Read the model definition and answer for the solid it produces. Units are mm, in the model's axes. Face numbers are marked on the shaded views. A direction names the side the tool comes from. Coordinates: 2 decimals unless noted, no trailing zeros. Loops run counter-clockwise (first coordinate to the right, second up) from the corner with the lowest first, then second, coordinate; pieces in that order, holes last.
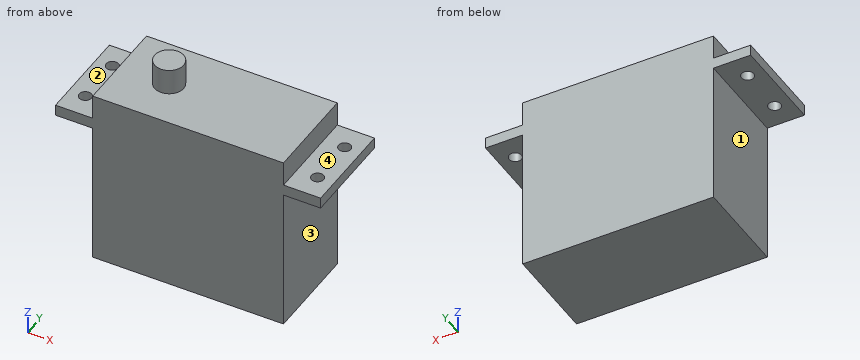
from build123d import *

# Parameters (mm, degrees)
SKETCH1_W                        = 54.356
SKETCH1_H                        = 19.685
EXTRUDE1_DEPTH                   = 42.2656
SKETCH3_OUTSIDE_W                = 70.678
SKETCH3_OUTSIDE_H                = 36.007
SKETCH3_OUTSIDE_R                = 2.9718
EXTRUDE2_DEPTH                   = 5.334
SKETCH7_W                        = 7.62
SKETCH7_H                        = 20.335773086
SKETCH7_H_2                      = 19.919316746
EXTRUDE4_DEPTH                   = 10.414
SKETCH8_W                        = 7.62
SKETCH8_H                        = 19.792977092
SKETCH8_H_2                      = 19.986836906
EXTRUDE5_DEPTH                   = 29.5656
F_39_0_0995_DIAMETER_HOLE1_D     = 2.5273
F_39_0_0995_DIAMETER_HOLE1_DEPTH = 12.7
F_39_0_0995_DIAMETER_HOLE1_TIP   = 0.759277521


with BuildPart() as part:
    # Sketch1 → Extrude1 (new body)
    with BuildSketch(Plane.XY):
        Rectangle(SKETCH1_W, SKETCH1_H)
    extrude(amount=EXTRUDE1_DEPTH)

    # Sketch3 outside → Extrude2 (cut)
    with BuildSketch(Plane.XY.offset(42.2656)):
        with Locations((0, 0.0005)):
            Rectangle(SKETCH3_OUTSIDE_W, SKETCH3_OUTSIDE_H)
        with Locations((-9.398, 0)):
            Circle(SKETCH3_OUTSIDE_R, mode=Mode.SUBTRACT)
    extrude(amount=-EXTRUDE2_DEPTH, mode=Mode.SUBTRACT)

    # Sketch7 → Extrude4 (cut)
    with BuildSketch(Plane.XY.offset(42.2656)):
        with Locations((23.368, 0)):
            Rectangle(SKETCH7_W, SKETCH7_H)
        with Locations((-23.368, 0)):
            Rectangle(SKETCH7_W, SKETCH7_H_2)
    extrude(amount=-EXTRUDE4_DEPTH, mode=Mode.SUBTRACT)

    # Sketch8 → Extrude5 (cut)
    with BuildSketch(Plane(origin=(0, 0, 0), x_dir=(-1, 0, 0), z_dir=(0, 0, -1))):
        with Locations((23.368, 0)):
            Rectangle(SKETCH8_W, SKETCH8_H)
        with Locations((-23.368, 0)):
            Rectangle(SKETCH8_W, SKETCH8_H_2)
    extrude(amount=-EXTRUDE5_DEPTH, mode=Mode.SUBTRACT)

    # #39 (0.0995) Diameter Hole1
    with Locations(Plane(origin=(-23.8125, 4.953, 31.8516), x_dir=(1, 0, 0), z_dir=(0, 0, 1))):
        with Locations((0, 0), (0, -9.906), (47.625, 0), (47.625, -9.906)):
            Hole(F_39_0_0995_DIAMETER_HOLE1_D / 2, depth=F_39_0_0995_DIAMETER_HOLE1_DEPTH)
            with Locations((0, 0, -(F_39_0_0995_DIAMETER_HOLE1_DEPTH + F_39_0_0995_DIAMETER_HOLE1_TIP / 2))):  # 118° drill point
                Cone(0, F_39_0_0995_DIAMETER_HOLE1_D / 2, F_39_0_0995_DIAMETER_HOLE1_TIP, mode=Mode.SUBTRACT)


solid = part.part
Q1. A cutting plane is placed at D-D (y = 7). Give the vertices of the cut face in (x, z).
Findings below:
outline: (-27.18, 29.57) - (-19.56, 29.57) - (-19.56, 0) - (19.56, 0) - (19.56, 29.57) - (27.18, 29.57) - (27.18, 31.85) - (19.56, 31.85) - (19.56, 36.93) - (-19.56, 36.93) - (-19.56, 31.85) - (-27.18, 31.85) - close
Q2. Which of the six approach directions +Z, -Z, +X, -X, +Y, -Y give full straight-line access (tool end or side, diameter ignored) to the marked faces 1, 2, 3 and 4?
Findings below:
face 1: -Z, -X, +Y, -Y
face 2: +Z, -X, +Y, -Y
face 3: -Z, +X, +Y, -Y
face 4: +Z, +X, +Y, -Y
Q3. Flat-ended cylindrical pins translate along their axes: pin 1 Ø1 at (y, z) = (-4.5, 35) entering from +X; pin 2 Ø3 at (x, y) = (-23.81, -4.95) entering from +Z; pin 3 Ø6 at (x, y) = (6.5, -3) entering from +Z. Find the tip coordinate at first contact, or state that the pin passes through.
Findings below:
pin 1: stops at x = 19.56
pin 2: stops at z = 31.85
pin 3: stops at z = 36.93
Q4. A cutting plane is placed at A-A (x = 23.5). Give the vertices of the cut face in (y, z), then the cut area to 3 significant figures.
Findings below:
outline: (-9.84, 29.57) - (-6.18, 29.57) - (-6.18, 31.85) - (-9.84, 31.85) - close; (-3.73, 29.57) - (3.73, 29.57) - (3.73, 31.85) - (-3.73, 31.85) - close; (6.18, 29.57) - (9.84, 29.57) - (9.84, 31.85) - (6.18, 31.85) - close
area: 33.8 mm2
Q5. A cutting plane is placed at B-B (y = 0). Give the vertices of the cut face in (x, z).
Findings below:
outline: (-27.18, 29.57) - (-19.56, 29.57) - (-19.56, 0) - (19.56, 0) - (19.56, 29.57) - (27.18, 29.57) - (27.18, 31.85) - (19.56, 31.85) - (19.56, 36.93) - (-6.43, 36.93) - (-6.43, 42.27) - (-12.37, 42.27) - (-12.37, 36.93) - (-19.56, 36.93) - (-19.56, 31.85) - (-27.18, 31.85) - close
Q6. Straight lines are drawn through the part: probe 1 along Z at (x, y) = (8, 2.5); probe 2 along X at (y, z) = (8.25, 10.5); probe 3 along Z at (x, y) = (21, -1). For each, find the intervals that lie inside material, in ascending order.
Findings below:
probe 1: z = 0 to 36.93
probe 2: x = -19.56 to 19.56
probe 3: z = 29.57 to 31.85
Q7. A cutting plane is placed at C-C (z = 39). Give the vertices of the cut face in (x, y), then the cut area to 3 significant figures.
Findings below:
outline: circle Ø5.94 at (-9.4, 0)
area: 27.7 mm2
